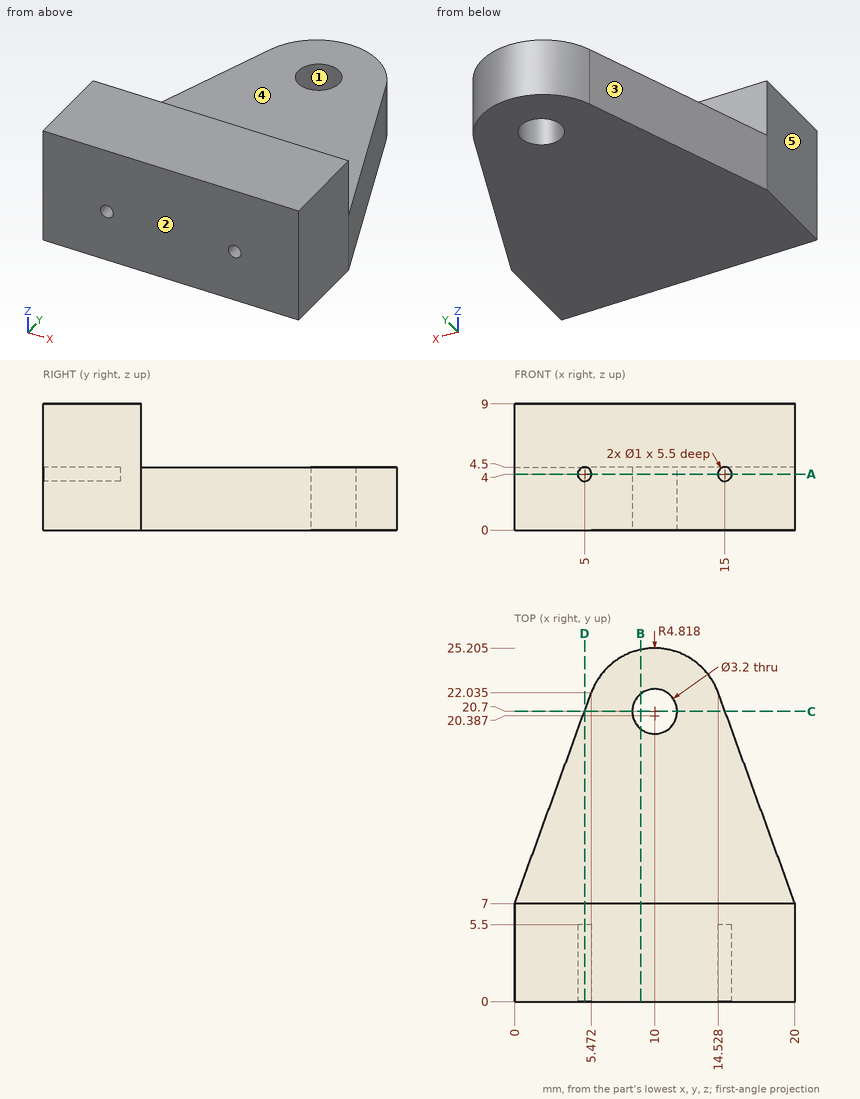
Geometry: see drawing. Coordinates: mm, zero at the bounding-box minimum. A direction names the side the tool comes from. Round coordinates to 2 decimals unless told otherwise and drop trailing zeros. Loops run counter-clockwise (first coordinate to the right, second up) from the corner with the lowest first, then second, coordinate; pieces in that order, holes last.
(1) Contact query for flat-ended pins moving along their axis: pin 1 Ø0.8 at (x, z) = (5, 4) entering from -Y; pin 2 Ø1.5 at (x, y) = (11.5, 15.5) entering from +Z; pin 3 Ø1.3 at (x, z) = (12.5, 6.5) entering from +Y. Output: stop coordinate, or through.
From the geometry:
pin 1: stops at y = 5.5
pin 2: stops at z = 4.5
pin 3: stops at y = 7
(2) Section query A-A (z = 4). Output: boundary loops of the cut face in (x, y) (1 decimal), and give its area (3 significant figures).
From the geometry:
outline: (0, 0) - (4.5, 0) - (4.5, 5.5) - (5.5, 5.5) - (5.5, 0) - (14.5, 0) - (14.5, 5.5) - (15.5, 5.5) - (15.5, 0) - (20, 0) - (20, 7) - (14.5, 22) arc R4.8 ccw to (5.5, 22) - (0, 7) - close; hole circle Ø3.2 at (10, 20.7)
area: 360 mm2
(3) Material intervals for probe 1 along Y at (x, z) = (10, 2.8) (1 decimal); probe 2 along Z at (x, y) = (15, 2.75); probe 3 along Z at (x, y) = (2.5, 9), sorted ascending.
From the geometry:
probe 1: y = 0 to 19.1, 22.3 to 25.2
probe 2: z = 0 to 3.5, 4.5 to 9
probe 3: z = 0 to 4.5
(4) Pull-direction query (Y, two-part tool) for the marked faces 1, 2 and 3; classes: +Y half, -Y half, draft (parallel to the pull), parting line (faces both ways), or undercut.
From the geometry:
face 1: undercut
face 2: -Y half
face 3: +Y half
(5) Section query C-C (y = 20.7). Output: boundary loops of the cut face in (x, z), and give its area (3 significant figures).
From the geometry:
outline: (4.99, 0) - (8.4, 0) - (8.4, 4.5) - (4.99, 4.5) - close; (11.6, 0) - (15.01, 0) - (15.01, 4.5) - (11.6, 4.5) - close
area: 30.7 mm2
(6) Section query B-B (x = 9). Output: boundary loops of the cut face in (y, z).
From the geometry:
outline: (0, 0) - (19.45, 0) - (19.45, 4.5) - (7, 4.5) - (7, 9) - (0, 9) - close; (21.95, 0) - (25.1, 0) - (25.1, 4.5) - (21.95, 4.5) - close
(7) Section query D-D (x = 5). Output: boundary loops of the cut face in (y, z).
From the geometry:
outline: (0, 0) - (20.74, 0) - (20.74, 4.5) - (7, 4.5) - (7, 9) - (0, 9) - (0, 4.5) - (5.5, 4.5) - (5.5, 3.5) - (0, 3.5) - close
(8) Access query for the marked faces 4 and 5. Directions: +Z, -Z, +X, -X, +Y, -Y. A direction counts if a zero-diameter tool reaches every point of the face in a straight line with its end or side. Return the directions, or none.
From the geometry:
face 4: +Z, +X, -X, +Y
face 5: +Z, -Z, -X, +Y, -Y
